Part model, mm, in its own coordinate system. A direction names the side the tool comes from. Coordinates: 2 decimals unless noted, no trailing zeros. Order: outer loops, then holes, each group sorted by start corner. A loop starts at its lowest first (then second) coordinate and runs counter-clockwise, first axis right, second up.
1) Cut at A-A (y = 0). List the corners of the cut face in (x, z).
2) Pin check, flat tip, straight feed: pin 1 Ø5.5 at (x, y) = (-1, -3.5) entering from +Z. Stop position of the tip, or through.
3) Cut at B-B (z = 16.25). List the corners of the cut face in (x, y), and give its area (3 significant figures).
4) Wall check: L1, parallel to X at y = -7, z = 11.75; L2, parallel to Z at x = 8, y = -12.5; L3, parallel to Y at x = -7.5, z = 18.25. Give the ranges that are in metal, low to high.
5) Mould opens along X. For faces 1 (the flat face through (-17.5, -2, 10)), 2 (the flat face through (-1, 13, 20)), 3 (the cylindrical face through (11.6, 11.64, 11.62)), 4 (the flat face through (0, -4, 0)) say: +X half, -X half, draft (parallel to the pull), parting line (faces both ways), or undercut.
6) Tool access for faces 5 (the cylindrical face through (-11.64, -3.81, 0.9)), 6 (the flat face through (17.5, -3, 10)): list every direction of +Z, -Z, +X, -X, +Y, -Y with a clear straight run to the whole face (end or side of a thin tool).
```python
from build123d import *

# Parameters (mm, degrees)
F1_DEPTH = 20
F0_W     = 25
F0_H     = 30
F2_DEPTH = 5
F3_R     = 4.99999
F4_R     = 3


# Not quite as in the source:
# - a fillet or chamfer is up to 0.001 mm smaller than in the source, because OpenCascade refuses the exact size


with BuildPart() as f1:
    # F0 (on Top) → F1 (new body)
    with BuildSketch(Plane.XY):
        with BuildLine():
            Line((12.5, -17.5), (17.5, -17.5))
            Line((17.5, -17.5), (17.5, 12.5))
            ThreePointArc((17.5, 12.5), (16.0355339059, 16.0355339059), (12.5, 17.5))
            Line((12.5, 17.5), (-12.5, 17.5))
            ThreePointArc((-12.5, 17.5), (-16.0355339059, 16.0355339059), (-17.5, 12.5))
            Line((-17.5, 12.5), (-17.5, -17.5))
            Line((-17.5, -17.5), (-12.5, -17.5))
            Line((-12.5, -17.5), (-12.5, 12.5))
            Line((-12.5, 12.5), (12.5, 12.5))
            Line((12.5, 12.5), (12.5, -17.5))
        make_face()
    extrude(amount=F1_DEPTH)

    # F0 (on Top) → F2 (join)
    with BuildSketch(Plane.XY):
        with Locations((0, -2.5)):
            Rectangle(F0_W, F0_H)
        with BuildLine():
            Line((12.5, -17.5), (17.5, -17.5))
            Line((17.5, -17.5), (17.5, 12.5))
            ThreePointArc((17.5, 12.5), (16.0355339059, 16.0355339059), (12.5, 17.5))
            Line((12.5, 17.5), (-12.5, 17.5))
            ThreePointArc((-12.5, 17.5), (-16.0355339059, 16.0355339059), (-17.5, 12.5))
            Line((-17.5, 12.5), (-17.5, -17.5))
            Line((-17.5, -17.5), (-12.5, -17.5))
            Line((-12.5, -17.5), (-12.5, 12.5))
            Line((-12.5, 12.5), (12.5, 12.5))
            Line((12.5, 12.5), (12.5, -17.5))
        make_face()
    extrude(amount=-F2_DEPTH)

    # F3 (radius 5 in the source; OpenCascade refuses exactly that, so slightly less here)
    f3_edges = [f1.edges().sort_by_distance(p)[0] for p in [
        (17.5, -2.5, -5),
        (16.035534, 16.035534, -5),
        (0, 17.5, -5),
        (-16.035534, 16.035534, -5),
        (-17.5, -2.5, -5),
        (0, -17.5, -5),
    ]]
    fillet(f3_edges, radius=F3_R)

    # F4
    f4_edges = [f1.edges().sort_by_distance(p)[0] for p in [
        (12.5, -2.5, 0),
        (-12.5, -2.5, 0),
        (12.5, 12.5, 10),
        (-12.5, 12.5, 10),
        (0, 12.5, 0),
    ]]
    fillet(f4_edges, radius=F4_R)


solid = f1.part
```
Geometry check:
1. outline: (-17.5, 0) arc R5 ccw to (-12.5, -5) - (12.5, -5) arc R5 ccw to (17.5, 0) - (17.5, 20) - (12.5, 20) - (12.5, 3) arc R3 cw to (9.5, 0) - (-9.5, 0) arc R3 cw to (-12.5, 3) - (-12.5, 20) - (-17.5, 20) - close
2. pin 1: stops at z = 0
3. outline: (-17.5, -17.5) - (-12.5, -17.5) - (-12.5, 9.5) arc R3 cw to (-9.5, 12.5) - (9.5, 12.5) arc R3 cw to (12.5, 9.5) - (12.5, -17.5) - (17.5, -17.5) - (17.5, 12.5) arc R5 ccw to (12.5, 17.5) - (-12.5, 17.5) arc R5 ccw to (-17.5, 12.5) - close
3. area: 468 mm2
4. L1: x = -17.5 to -12.5, 12.5 to 17.5
4. L2: z = -5 to 0
4. L3: y = 12.5 to 17.5
5. face 1: -X half
5. face 2: draft
5. face 3: undercut
5. face 4: undercut
6. face 5: +Z, -Y
6. face 6: +Z, -Z, +X, +Y, -Y
